Here's how the part is built. I have some questions about the finished solid (model axes, mm). A direction names the side the tool comes from. Round coordinates to 2 decimals unless told otherwise and drop trailing zeros. Write each loop counter-clockwise with the first axis right and the second up, starting at its lowest first coordinate (ties: lowest second). Pieces come first, ordered by that corner, then holes. Notation, with made-up numbers: (12, 41.5) -> (49, 41.5) arc R19 cw to (49, 67.5) -> close; hole circle Ø3 at (89.25, 56). An arc over 180 degrees is marked (long way). Put each result on its own line as item: value. Start each with the question number.
1. Suppose I cut it at C-C (x = 179). Please give me the cut outline in (y, z), then the cut area to 3 significant figures.
2. I need wall thicknesses on probe 1 along Y at (x, z) = (387.5, 2.75); probe 2 along Y at (x, z) = (70, 6.5); probe 3 along Y at (x, z) = (435.5, 3.5). Which ranges of each line are inside material? Lowest first, please. Write a range as from..to.
3. For pin 1 (4 mm diameter, centred on y = 673.5, z = 2, fed in from +X); pin 2 (1 mm diameter, centred on x = 322.5, z = 3, fed in from +Y), each with a flat end and sliding along its axis, tell me the tip position at first contact or that it passes through.
4. Suppose I cut it at A-A (z = 3.75). Please give me the cut outline in (x, y).
5. Suppose I cut it at B-B (y = 669.5). Please give me the cut outline in (x, z).
6. We'd pull the mould along Y, two halves only. Please class faces 4 (the face through (418.326, 668.49, 3.944)), 5 (the face through (421.38, 679.57, 3.94)), 6 (the face through (297, 298, 8)): +Y half, -Y half, draft (parallel to the pull), parting line (faces both ways), or undercut.
7. Which directions (+Z, -Z, +X, -X, +Y, -Y) give clear straight access to the entire face, cutting with the end or side of a thin tool? Please do faces 1 (the face through (297, 298, 0)), 2 (the face through (372.07, 578.88, 3.94)), 3 (the face through (413.5, 662, 3.9)).
8. Suppose I cut it at D-D (y = 373.5). Please give me the cut outline in (x, z), then the cut area to 3 significant figures.
```python
from build123d import *

# Parameters (mm, degrees)
SKETCH1_W           = 8
SKETCH1_H           = 113.93
BOSS_EXTRUDE1_DEPTH = 8


with BuildPart() as part:
    # Sketch1 → Boss-Extrude1 (new body)
    with BuildSketch(Plane.XY):
        Polygon((0, 192), (0, 0), (492, 0), (492, 608.949580676), (348.752525317, 752.197055359), (348.752525317, 602.197055359), (396.053847577, 554.895733099), (401.154700619, 563.730669729), (403.75277683, 562.230669729), (398.25, 552.699580676), (190, 192), align=None)
        with Locations((362.728293748, 663.1220766)):
            Rectangle(SKETCH1_W, SKETCH1_H, mode=Mode.SUBTRACT)
        Polygon((394.083632807, 570.801737541), (376.405963277, 588.479407071), (382.062817527, 594.13626132), (399.740487057, 576.458591791), align=None, mode=Mode.SUBTRACT)
        Polygon((443.916069982, 631.585591867), (382.284642934, 693.217018915), (387.941497183, 698.873873165), (449.572924232, 637.242446117), align=None, mode=Mode.SUBTRACT)
    extrude(amount=BOSS_EXTRUDE1_DEPTH)


solid = part.part
```
Verdict:
1. outline: (0, 0) -> (192, 0) -> (192, 8) -> (0, 8) -> close
1. area: 1,540 mm^2
2. probe 1: y = 0..534.08, 563.45..577.39, 588.7..688, 698.43..713.45
2. probe 2: y = 0..192
2. probe 3: y = 0..640, 651.32..665.45
3. pin 1: stops at x = 429.45
3. pin 2: stops at y = 422.36
4. outline: (0, 0) -> (492, 0) -> (492, 608.95) -> (348.75, 752.2) -> (348.75, 602.2) -> (396.05, 554.9) -> (401.15, 563.73) -> (403.75, 562.23) -> (190, 192) -> (0, 192) -> close; hole (358.73, 606.16) -> (366.73, 606.16) -> (366.73, 720.09) -> (358.73, 720.09) -> close; hole (376.41, 588.48) -> (394.08, 570.8) -> (399.74, 576.46) -> (382.06, 594.14) -> close; hole (382.28, 693.22) -> (443.92, 631.59) -> (449.57, 637.24) -> (387.94, 698.87) -> close
5. outline: (348.75, 0) -> (358.73, 0) -> (358.73, 8) -> (348.75, 8) -> close; (366.73, 0) -> (406, 0) -> (406, 8) -> (366.73, 8) -> close; (417.32, 0) -> (431.45, 0) -> (431.45, 8) -> (417.32, 8) -> close
6. face 4: undercut
6. face 5: +Y half
6. face 6: draft
7. face 1: -Z, +X, -X, +Y, -Y
7. face 2: +Z, -Z, -X
7. face 3: +Z, -Z
8. outline: (294.79, 0) -> (492, 0) -> (492, 8) -> (294.79, 8) -> close
8. area: 1,580 mm^2
